Could you check a few things on this model? Use its own coordinates, in mm. Face numbers are marked on the shaded views. A direction names the side the tool comes from. Coordinates: 2 decimals unless noted, no trailing zeros. Write each loop counter-clockwise with the first axis right and the second up, starting at its lowest first coordinate (ties: lowest second). Pieces come first, ordered by that corner, then holes. Notation, with made-up numbers: (-22.5, 10.5) - (30.5, 10.5) arc R25 ccw to (30.5, 25.5) - close; hole circle Ø8 at (-1.5, 24.5). An arc over 180 degrees is marked (long way). Answer as a JSON object with one key per item and string values. Group by question number.
1) On a 3-axis mill with a long thin cutter (end or side, diameter ignored), from which of +Z, -Z, +X, -X, +Y, -Y can I reach the whole of each face in a straight line? I mean the marked faces 4 and 5. Say none if no direction works.
2) If we section it at A-A (z = 13): Write out the boundary of the cut face in (x, y).
3) We'd pull the mould along X, two halves only. Please class the marked faces 1, 2 and 3: released by +X, released by -X, zero draft, split by the parting line, or undercut.
4) If we section it at D-D (z = -10): Write out the boundary of the cut face in (x, y).
5) Will these pins go through, and if not, where does the flat tip stop? pin 1 Ø5 at (y, z) = (-46, 21.5) entering from +X; pin 2 Ø4 at (x, z) = (5, -13) entering from +Y; pin 3 Ø13 at (x, z) = (-2, -10.5) entering from -Y.
6) If we section it at B-B (x = 5): Write out the boundary of the cut face in (y, z), plus the area to 3 significant figures.
7) If we section it at C-C (z = 21.5): Write out the boundary of the cut face in (x, y).
8) Please list where these lines run through material, in increasing order: line 1 along Z through (x, y) = (5, 1); line 2 along Z through (x, y) = (-13.8, -46); line 3 along X through (y, z) = (-16, 21).
```python
from build123d import *

# Parameters (mm, degrees)
F0_R         = 2.25
F0_W         = 4
F0_H         = 20
F1_DEPTH     = 4
F2_W         = 4
F2_H         = 20
F3_DEPTH     = 49
F5_DEPTH     = 13.2825661727
F6_T1_DEPTH  = 4.75
F6_T3_DEPTH  = 48.5
F6_T5_DEPTH  = 25.5
F6_T7_DEPTH  = 49
F6_T9_DEPTH  = 4.75
F6_T11_DEPTH = 7.7618980501
F6_S15_W     = 0.51
F6_S15_H     = 0.51
F6_T16_DEPTH = 0.51
F6_S21_W     = 0.51
F6_S21_H     = 0.51
F6_T22_DEPTH = 0.51
F6_S27_W     = 0.51
F6_S27_H     = 0.51
F6_T28_DEPTH = 0.51
F6_T34_DEPTH = 16.75
F6_T39_DEPTH = 20.75
F6_T45_DEPTH = 49.75
F6_T49_DEPTH = 26.75
F7_R         = 1.5
F8_DEPTH     = 30.001


# Not quite as in the source:
# - a fillet or chamfer that OpenCascade refuses, or shapes differently, is made with other operations: its cross-section is extruded or revolved along the edge and cut away or added


with BuildPart() as f1:
    # F0 (on Front) → F1 (new body)
    with BuildSketch(Plane.XZ):
        Polygon((15, 25), (-11, 25), (-11, 5), (-1, -25), (15, -25), align=None)
        with Locations((5, -13)):
            Circle(F0_R, mode=Mode.SUBTRACT)
        with Locations((5, 13)):
            Circle(F0_R, mode=Mode.SUBTRACT)
        with Locations((-13, 15)):
            Rectangle(F0_W, F0_H)
        Polygon((-11, 5), (-15, 5), (-5, -25), (-1, -25), align=None)
    extrude(amount=-F1_DEPTH)

    # F2 (on face) → F3 (join)
    with BuildSketch(Plane.XZ):
        with Locations((-13, 15)):
            Rectangle(F2_W, F2_H)
        Polygon((-11, 5), (-15, 5), (-5, -25), (-1, -25), align=None)
    extrude(amount=F3_DEPTH)

    # F4 (on face) → F5 (cut, through all)
    with BuildSketch(Plane(origin=(-8.4, 0, -2.8), x_dir=(0, 1, 0), z_dir=(0.9486832981, 0, 0.316227766))):
        Polygon((0, -23.4008546852), (-49, 8.2219219164), (-49, -23.4008546852), align=None)
    extrude(amount=-F5_DEPTH, mode=Mode.SUBTRACT)

    # F6: fillet of radius 0.5 on 9 edges, made by hand

    # F6_s2 → F6_t1 (cut)
    with BuildSketch(Plane.YZ.offset(-16.25)):
        with BuildLine():
            ThreePointArc((-48.5, 25), (-48.8535533906, 24.8535533906), (-49, 24.5))
            Line((-49, 24.5), (-49, 25))
            Line((-49, 25), (-48.5, 25))
        make_face()
    extrude(amount=F6_T1_DEPTH, mode=Mode.SUBTRACT)

    # F6_s4 → F6_t3 (cut)
    with BuildSketch(Plane.XZ):
        with BuildLine():
            ThreePointArc((-11.5, 25), (-11.1464466094, 24.8535533906), (-11, 24.5))
            Line((-11, 24.5), (-11, 25))
            Line((-11, 25), (-11.5, 25))
        make_face()
    extrude(amount=F6_T3_DEPTH, mode=Mode.SUBTRACT)

    # F6_s6 → F6_t5 (cut)
    with BuildSketch(Plane.YZ.offset(-11)):
        with BuildLine():
            ThreePointArc((0.5, 25), (0.1464466094, 24.8535533906), (0, 24.5))
            Line((0, 24.5), (0, 25))
            Line((0, 25), (0.5, 25))
        make_face()
    extrude(amount=F6_T5_DEPTH, mode=Mode.SUBTRACT)

    # F6_s8 → F6_t7 (cut)
    with BuildSketch(Plane.XY.offset(-24.5)):
        with BuildLine():
            ThreePointArc((15, 0.5), (14.8535533906, 0.1464466094), (14.5, 0))
            Line((14.5, 0), (15, 0))
            Line((15, 0), (15, 0.5))
        make_face()
    extrude(amount=F6_T7_DEPTH, mode=Mode.SUBTRACT)

    # F6_s10 → F6_t9 (cut)
    with BuildSketch(Plane.XZ.offset(-5.25)):
        with BuildLine():
            ThreePointArc((14.5, 25), (14.8535533906, 24.8535533906), (15, 24.5))
            Line((15, 24.5), (15, 25))
            Line((15, 25), (14.5, 25))
        make_face()
        with BuildLine():
            ThreePointArc((15, -24.5), (14.8535533906, -24.8535533906), (14.5, -25))
            Line((14.5, -25), (15, -25))
            Line((15, -25), (15, -24.5))
        make_face()
    extrude(amount=F6_T9_DEPTH, mode=Mode.SUBTRACT)

    # F6_s12 → F6_t11 (cut)
    with BuildSketch(Plane.XZ.offset(-4.9009490251)):
        with BuildLine():
            ThreePointArc((-4.63962039, -25), (-4.9319755323, -24.9056210926), (-5.113962039, -24.658113883))
            Line((-5.113962039, -24.658113883), (-5, -25))
            Line((-5, -25), (-4.63962039, -25))
        make_face()
    extrude(amount=F6_T11_DEPTH, mode=Mode.SUBTRACT)


with BuildPart() as f6_tool14:
    # F6_s15 → F6_t16 (new body)
    with BuildSketch(Plane.XY.offset(24.5)):
        with Locations((-11.245, -48.755)):
            Rectangle(F6_S15_W, F6_S15_H)
    extrude(amount=F6_T16_DEPTH)

    # F6_s17 → F6_t18 (revolve, cut)
    with BuildSketch(Plane(origin=(-11.5, -48.5, 24.5), x_dir=(-0.7071067812, 0.7071067812, 0), z_dir=(0.7071067812, 0.7071067812, 0))):
        with BuildLine():
            ThreePointArc((0, -0.5), (0.5, 0), (0, 0.5))
            Line((0, 0.5), (0, -0.5))
        make_face()
    revolve(axis=Axis((-11.5, -48.5, 24.5), (0, 0, 1)), mode=Mode.SUBTRACT)


with BuildPart() as f1_1:
    add(f1.part)

    # F6_t13: cut F6_tool14
    add(f6_tool14.part, mode=Mode.SUBTRACT)


with BuildPart() as f6_tool20:
    # F6_s21 → F6_t22 (new body)
    with BuildSketch(Plane.XY.offset(24.5)):
        with Locations((14.755, 0.245)):
            Rectangle(F6_S21_W, F6_S21_H)
    extrude(amount=F6_T22_DEPTH)

    # F6_s23 → F6_t24 (revolve, cut)
    with BuildSketch(Plane(origin=(14.5, 0.5, 24.5), x_dir=(-0.7071067812, 0.7071067812, 0), z_dir=(0.7071067812, 0.7071067812, 0))):
        with BuildLine():
            ThreePointArc((0, -0.5), (0.5, 0), (0, 0.5))
            Line((0, 0.5), (0, -0.5))
        make_face()
    revolve(axis=Axis((14.5, 0.5, 24.5), (0, 0, 1)), mode=Mode.SUBTRACT)


with BuildPart() as f1_2:
    add(f1_1.part)

    # F6_t19: cut F6_tool20
    add(f6_tool20.part, mode=Mode.SUBTRACT)


with BuildPart() as f6_tool26:
    # F6_s27 → F6_t28 (new body)
    with BuildSketch(Plane.YZ.offset(14.5)):
        with Locations((0.245, -24.755)):
            Rectangle(F6_S27_W, F6_S27_H)
    extrude(amount=F6_T28_DEPTH)

    # F6_s29 → F6_t30 (revolve, cut)
    with BuildSketch(Plane(origin=(14.5, 0.5, -24.5), x_dir=(0, 0.7071067812, 0.7071067812), z_dir=(0, 0.7071067812, -0.7071067812))):
        with BuildLine():
            ThreePointArc((0, -0.5), (0.5, 0), (0, 0.5))
            Line((0, 0.5), (0, -0.5))
        make_face()
    revolve(axis=Axis((14.5, 0.5, -24.5), (1, 0, 0)), mode=Mode.SUBTRACT)


with BuildPart() as f1_3:
    add(f1_2.part)

    # F6_t25: cut F6_tool26
    add(f6_tool26.part, mode=Mode.SUBTRACT)


with BuildPart() as f6_tool32:
    # F6_s33 → F6_t34 (new body)
    with BuildSketch(Plane.YZ.offset(-2.25)):
        with BuildLine():
            ThreePointArc((0, -24.5), (0.1464466094, -24.8535533906), (0.5, -25))
            Line((0.5, -25), (0, -25))
            Line((0, -25), (0, -24.5))
        make_face()
    extrude(amount=F6_T34_DEPTH)

    split(bisect_by=Plane(origin=(-8.4, 0, -2.8), x_dir=(0, 1, 0), z_dir=(0.9486832981, 0, 0.316227766)), keep=Keep.TOP)


with BuildPart() as f1_4:
    add(f1_3.part)

    # F6_t31: cut F6_tool32
    add(f6_tool32.part, mode=Mode.SUBTRACT)


with BuildPart() as f6_tool37:
    # F6_s38 → F6_t39 (new body)
    with BuildSketch(Plane.XY.offset(3.75)):
        with BuildLine():
            ThreePointArc((-11.5, -49), (-11.1464466094, -48.8535533906), (-11, -48.5))
            Line((-11, -48.5), (-11, -49))
            Line((-11, -49), (-11.5, -49))
        make_face()
    extrude(amount=F6_T39_DEPTH)

    split(bisect_by=Plane(origin=(-8.4, 0, -2.8), x_dir=(0, 1, 0), z_dir=(0.9486832981, 0, 0.316227766)), keep=Keep.TOP)


with BuildPart() as f1_5:
    add(f1_4.part)

    # F6_t36: cut F6_tool37
    add(f6_tool37.part, mode=Mode.SUBTRACT)


with BuildPart() as f6_tool43:
    # F6_s44 → F6_t45 (new body)
    with BuildSketch(Plane.XZ.offset(-1.25)):
        with BuildLine():
            ThreePointArc((-11.5, 25), (-11.1464466094, 24.8535533906), (-11, 24.5))
            Line((-11, 24.5), (-11, 25))
            Line((-11, 25), (-11.5, 25))
        make_face()
    extrude(amount=F6_T45_DEPTH)

    split(bisect_by=Plane.XZ, keep=Keep.BOTTOM)


with BuildPart() as f6_tool47:
    # F6_s48 → F6_t49 (new body)
    with BuildSketch(Plane.YZ.offset(14.5)):
        with BuildLine():
            ThreePointArc((0.5, 25), (0.1464466094, 24.8535533906), (0, 24.5))
            Line((0, 24.5), (0, 25))
            Line((0, 25), (0.5, 25))
        make_face()
    extrude(amount=-F6_T49_DEPTH)

    split(bisect_by=Plane.YZ.offset(-11), keep=Keep.BOTTOM)


with BuildPart() as f6_tool43_1:
    add(f6_tool43.part)

    # F6_t51: intersect F6_tool47
    add(f6_tool47.part, mode=Mode.INTERSECT)


with BuildPart() as f1_6:
    add(f1_5.part)

    # F6_t41: cut F6_tool43
    add(f6_tool43_1.part, mode=Mode.SUBTRACT)

    # F7 (on face) → F8 (cut, through all)
    with BuildSketch(Plane(origin=(-15, 0, 0), x_dir=(0, -1, 0), z_dir=(-1, 0, 0))):
        with Locations((26.5, 21.5)):
            Circle(F7_R)
        with Locations((46, 21.5)):
            Circle(F7_R)
    extrude(amount=-F8_DEPTH, mode=Mode.SUBTRACT)


solid = f1_6.part
```
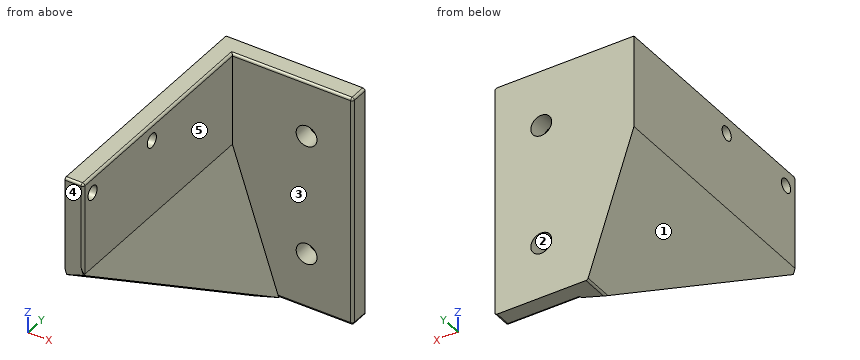
Here are the results:
{
 "1": {"face 4": "+Z, -Z, +X, -X, -Y", "face 5": "+Z, +X, -Y"},
 "2": {"outline": "(-15, -49) - (-11.5, -49) arc R0.5 ccw to (-11, -48.5) - (-11, 0) - (2.75, 0) - (2.75, 4) - (-15, 4) - close; (7.25, 0) - (14.5, 0) arc R0.5 ccw to (15, 0.5) - (15, 4) - (7.25, 4) - close"},
 "3": {"face 1": "released by -X", "face 2": "undercut", "face 3": "zero draft"},
 "4": {"outline": "(-10, -26.46) - (-6, -24.5) - (-6, 0) - (14.5, 0) arc R0.5 ccw to (15, 0.5) - (15, 4) - (-10, 4) - close"},
 "5": {"pin 1": "stops at x = -11", "pin 2": "passes through", "pin 3": "stops at y = -30.15"},
 "6": {"outline": "(0, -24.5) arc R0.5 ccw to (0.5, -25) - (4, -25) - (4, -15.25) - (0, -15.25) - close; (0, -10.75) - (4, -10.75) - (4, 10.75) - (0, 10.75) - close; (0, 15.25) - (4, 15.25) - (4, 25) - (0.5, 25) arc R0.5 ccw to (0, 24.5) - close", "area": "164 mm²"},
 "7": {"outline": "(-15, -49) - (-11.5, -49) arc R0.5 ccw to (-11, -48.5) - (-11, -47.5) - (-15, -47.5) - close; (-15, -44.5) - (-11, -44.5) - (-11, -28) - (-15, -28) - close; (-15, -25) - (-11, -25) - (-11, 0) - (14.5, 0) arc R0.5 ccw to (15, 0.5) - (15, 4) - (-15, 4) - close"},
 "8": {"line 1": "z = -25 to -15.25, -10.75 to 10.75, 15.25 to 25", "line 2": "z = 2.03 to 20, 23 to 25", "line 3": "x = -15 to -11"}
}
